Here's the drawing with two shaded views (mm, measured from the low corner). I have some questions. A direction names the side the tool comes from. Round coordinates to 2 decimals unless told otherwise and drop trailing zeros. Order: outer loops, then holes, each group sorted by start corner. A loop starts at its lowest first (then second) coordinate and runs counter-clockwise, first axis right, second up. Notation, with made-up numbers: (-0.5, 35) - (27.5, 35) arc R20 cw to (27.5, 62) - close; hole circle Ø2 at (65, 19.25). An arc over 180 degrees is marked (long way). One line per item, written item: value.
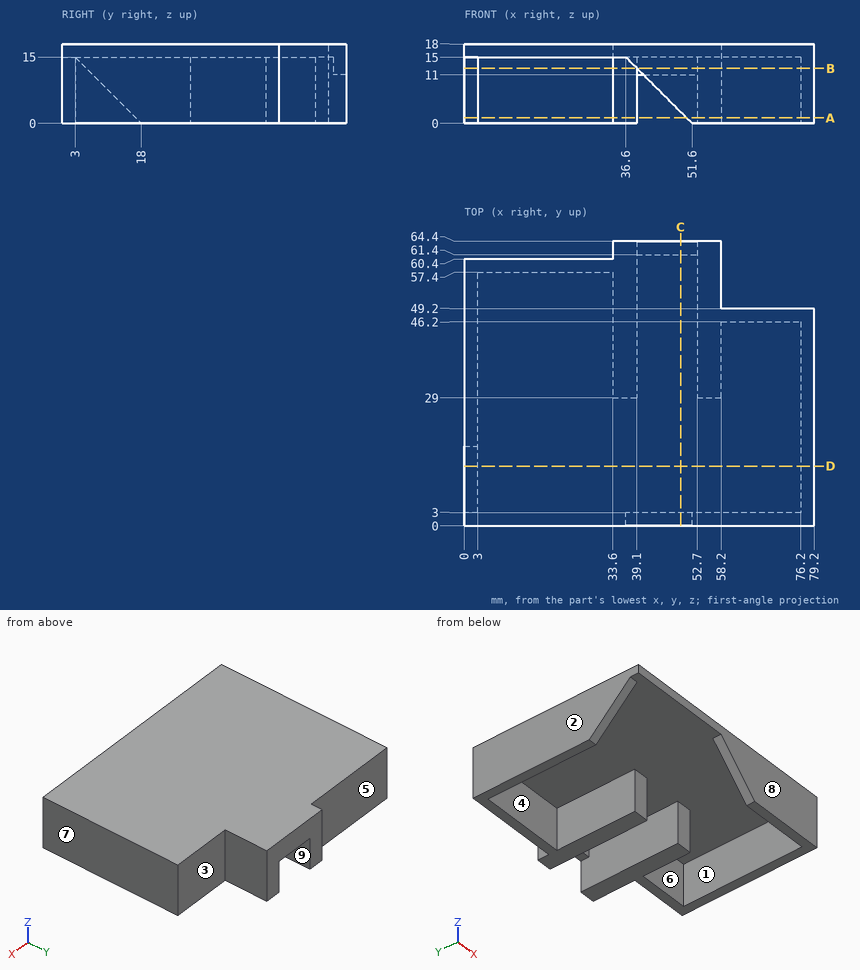
Q1. Which directions (+Z, -Z, +X, -X, +Y, -Y) give clear straight access to the entire face, cutting with the end or side of a thin tool? Please do the marked faces 1, 2, 3, 4 and 5.
Results list:
face 1: -Z
face 2: +Z, -Z, -X, +Y, -Y
face 3: +Z, -Z, +X, +Y
face 4: -Z, -Y
face 5: +Z, -Z, -X, +Y
Q2. If we section it at A-A, the plane z = 1.25: Please give me the cut outline in (x, y).
Results list:
outline: (0, 16.75) - (3, 16.75) - (3, 57.4) - (33.6, 57.4) - (33.6, 29) - (39.1, 29) - (39.1, 64.4) - (33.6, 64.4) - (33.6, 60.4) - (0, 60.4) - close; (50.35, 0) - (79.2, 0) - (79.2, 49.2) - (58.2, 49.2) - (58.2, 64.4) - (52.7, 64.4) - (52.7, 29) - (58.2, 29) - (58.2, 46.2) - (76.2, 46.2) - (76.2, 3) - (50.35, 3) - close
Q3. We'd pull the mould along Y, two halves only. Please class the marked faces 6, 7, 8 and 9: released by +Y, released by -Y, zero draft, split by the parting line, or undercut.
Results list:
face 6: undercut
face 7: zero draft
face 8: released by -Y
face 9: undercut
Q4. If we section it at D-D, the plane y = 13.5: Please give me the cut outline in (x, z).
Results list:
outline: (0, 4.5) - (3, 4.5) - (3, 15) - (76.2, 15) - (76.2, 0) - (79.2, 0) - (79.2, 18) - (0, 18) - close
Q5. If I drill on line 1 along X through (y, z) = (31, 5.75); line 2 along X through (y, z) = (53.5, 1.25); line 3 along Y through (x, z) = (73.5, 1), over which ranges is the centre line in solid material (lowest first)?
Results list:
line 1: 0 to 3, 33.6 to 39.1, 52.7 to 58.2, 76.2 to 79.2
line 2: 0 to 3, 33.6 to 39.1, 52.7 to 58.2
line 3: 0 to 3, 46.2 to 49.2
Q6. If we section it at B-B, the plane z = 12.5: Please give me the cut outline in (x, y).
Results list:
outline: (0, 5.5) - (3, 5.5) - (3, 57.4) - (33.6, 57.4) - (33.6, 29) - (39.1, 29) - (39.1, 61.4) - (52.7, 61.4) - (52.7, 29) - (58.2, 29) - (58.2, 46.2) - (76.2, 46.2) - (76.2, 3) - (39.1, 3) - (39.1, 0) - (79.2, 0) - (79.2, 49.2) - (58.2, 49.2) - (58.2, 64.4) - (33.6, 64.4) - (33.6, 60.4) - (0, 60.4) - close
Q7. If we section it at C-C, the plane x = 49: Please give me the cut outline in (y, z), then the cut area to 3 significant figures.
Results list:
outline: (0, 2.6) - (3, 2.6) - (3, 15) - (61.4, 15) - (61.4, 11) - (64.4, 11) - (64.4, 18) - (0, 18) - close
area: 242 mm²
Q8. Will these pins go through, and if not, where does the flat tip stop? pin 1 (1 mm diameter, centred on x = 61.5, z = 4, fed in from +Y); pin 2 (9 mm diameter, centred on x = 8.5, z = 6.5, fed in from +Y); pin 3 (4.5 mm diameter, centred on y = 23, z = 5, fed in from -X); pin 4 (1.6 mm diameter, centred on x = 35.5, z = 4.5, fed in from -Y).
Results list:
pin 1: y = 49.2
pin 2: y = 60.4
pin 3: x = 0
pin 4: y = 29
